from build123d import *

# Parameters (mm, degrees)
SKETCH1_W           = 136.4
SKETCH1_H           = 136.4
BOSS_EXTRUDE1_DEPTH = 3.175
BOSS_EXTRUDE2_DEPTH = 3.175
CUT_EXTRUDE2_DEPTH  = 111.78755853
CIRPATTERN1_COUNT   = 4


with BuildPart() as part:
    # Sketch1 → Boss-Extrude1 (new body)
    with BuildSketch(Plane(origin=(0, 0, 0), x_dir=(1, 0, 0), z_dir=(0, 1, 0))):
        Rectangle(SKETCH1_W, SKETCH1_H)
    extrude(amount=BOSS_EXTRUDE1_DEPTH)

    # Sketch2 → Boss-Extrude2 (add)
    with BuildSketch(Plane(origin=(0, 0, 0), x_dir=(1, 0, 0), z_dir=(0, 1, 0))):
        with BuildLine():
            Line((-68.2, 43.625), (-68.2, 24.575))
            ThreePointArc((-68.2, 24.575), (-71.490806564, 29.899636871), (-77.725, 29.3375))
            ThreePointArc((-77.725, 29.3375), (-83.959193436, 28.775363129), (-87.25, 34.1))
            ThreePointArc((-87.25, 34.1), (-83.959193436, 39.424636871), (-77.725, 38.8625))
            ThreePointArc((-77.725, 38.8625), (-71.490806564, 38.300363129), (-68.2, 43.625))
        make_face()
    boss_extrude2 = extrude(amount=BOSS_EXTRUDE2_DEPTH)

    # Sketch2<3> → Cut-Extrude2 (cut, through all)
    with BuildSketch(Plane(origin=(0, 0, 0), x_dir=(1, 0, 0), z_dir=(0, 1, 0))):
        with BuildLine():
            Line((-68.2, -43.625), (-68.2, -24.575))
            ThreePointArc((-68.2, -24.575), (-64.909193436, -29.899636871), (-58.675, -29.3375))
            ThreePointArc((-58.675, -29.3375), (-52.440806564, -28.775363129), (-49.15, -34.1))
            ThreePointArc((-49.15, -34.1), (-52.440806564, -39.424636871), (-58.675, -38.8625))
            ThreePointArc((-58.675, -38.8625), (-64.909193436, -38.300363129), (-68.2, -43.625))
        make_face()
    cut_extrude2 = extrude(amount=CUT_EXTRUDE2_DEPTH, mode=Mode.SUBTRACT)

    # CirPattern1: Boss-Extrude2, Cut-Extrude2 ×4 about axis
    cirpattern1_axis = Axis((0, 0, 0), (0, 1, 0))
    add([boss_extrude2.rotate(cirpattern1_axis, i * 360 / CIRPATTERN1_COUNT) for i in range(1, CIRPATTERN1_COUNT)])
    add([cut_extrude2.rotate(cirpattern1_axis, i * 360 / CIRPATTERN1_COUNT) for i in range(1, CIRPATTERN1_COUNT)], mode=Mode.SUBTRACT)


solid = part.part
Verification items for the finished model (mm, model axes). Coordinates: 2 decimals unless noted, no trailing zeros. Order: outer loops, then holes, each group sorted by start corner. A loop starts at its lowest first (then second) coordinate and runs counter-clockwise, first axis right, second up. Notation, with made-up numbers: M 46.5,54 L 79.5,54 A30 cw 79.5,82 Z; hole C 33.5,25.5 d10. An arc over 180 degrees is marked long. One line per item, written item: value. Start each with the question number.
Item 1: Sectioned sample at C-C (x = 7). Enter the section's corners in (y, z) (3 decimals), then the cut area to 3 significant figures.
Item 2: Scan lines: probe 1 along Z at (x, y) = (29, 0.6); probe 2 along X at (y, z) = (2.1, 29); probe 3 along Z at (x, y) = (-74, 0.7). Record each from-to range of solid material in increasing order.
Item 3: Sectioned sample at A-A (x = 65.5). Enter the section's corners in (y, z) (3 decimals), then the cut area to 3 significant figures.
Item 4: Gauge pin test, flat ends, axial feed: pin 1 (5 mm diameter, centred on x = 46, z = 60.5, fed in from -Y); pin 2 (1 mm diameter, centred on y = 2, z = 61.5, fed in from +X); pin 3 (1.6 mm diameter, centred on x = -61, y = 1, fed in from -Z); pin 4 (1.6 mm diameter, centred on y = 1.5, z = -60, fed in from -X). Record the tip position at first contact, or that the pin passes through.
Item 5: Sectioned sample at B-B (z = -62). Enter the section's corners in (x, y) (3 decimals), then the cut area to 3 significant figures.
Item 6: Sectioned sample at D-D (z = 10.5). Enter the section's corners in (x, y) (3 decimals).
Conclusion:
1. outline: M 0,-68.2 L 3.175,-68.2 L 3.175,68.2 L 0,68.2 Z
1. area: 433 mm^2
2. probe 1: z = -84.37 to -78.23, -70.17 to 52.03, 58.17 to 66.23
2. probe 2: x = -66.23 to -58.17, -52.03 to 70.17, 78.23 to 84.37
2. probe 3: z = -37.67 to -30.53
3. outline: M 0,-68.2 L 3.175,-68.2 L 3.175,-38.639 L 0,-38.639 Z; M 0,-29.561 L 3.175,-29.561 L 3.175,68.2 L 0,68.2 Z
3. area: 404 mm^2
4. pin 1: stops at y = 0
4. pin 2: stops at x = 68.2
4. pin 3: stops at z = -68.2
4. pin 4: stops at x = -68.2
5. outline: M -68.2,0 L -37.677,0 L -37.677,3.175 L -68.2,3.175 Z; M -30.523,0 L 68.2,0 L 68.2,3.175 L -30.523,3.175 Z
5. area: 410 mm^2
6. outline: M -68.2,0 L 68.2,0 L 68.2,3.175 L -68.2,3.175 Z
